```python
from build123d import *

# Parameters (mm, degrees)
CUT_EXTRUDE1_DEPTH = 101.6
SKETCH3_R          = 3.175
CUT_EXTRUDE2_DEPTH = 12.7


with BuildPart() as part:
    # Sketch1 → Revolve1 (revolve)
    with BuildSketch(Plane.XY):
        Polygon((0, 0), (27.94, 0), (27.94, 7.9375), (19.05, 7.9375), (19.05, 19.84375), (31.75, 19.84375), (31.75, 22.621875), (22.225, 22.621875), (22.225, 51.196875), (17.2640625, 51.196875), (17.2640625, 54.371875), (0, 54.371875), align=None)
    revolve(axis=Axis((0, 0, 0), (0, 1, 0)))

    # Sketch2 → Cut-Extrude1 (cut)
    with BuildSketch(Plane.XZ):
        Polygon((12.7, 7.332348419), (0, 14.664696837), (-12.7, 7.332348419), (-12.7, -7.332348419), (0, -14.664696837), (12.7, -7.332348419), align=None)
    extrude(amount=-CUT_EXTRUDE1_DEPTH, mode=Mode.SUBTRACT)

    # Sketch3 → Cut-Extrude2 (cut)
    with BuildSketch(Plane.XZ):
        with Locations((0, 22.225)):
            Circle(SKETCH3_R)
        with Locations((19.247414599, -11.1125)):
            Circle(SKETCH3_R)
        with Locations((-19.247414599, -11.1125)):
            Circle(SKETCH3_R)
    extrude(amount=-CUT_EXTRUDE2_DEPTH, mode=Mode.SUBTRACT)


solid = part.part
```
Geometry: final body of the model. Coordinates: model frame, mm. A direction names the side the tool comes from. Coordinates: 2 decimals unless noted, no trailing zeros. Order: outer loops, then holes, each group sorted by start corner. A loop starts at its lowest first (then second) coordinate and runs counter-clockwise, first axis right, second up.
Item 1: Section query D-D (z = 21). Output: boundary loops of the cut face in (x, y).
Answer:
outline: (-23.81, 19.84) - (23.81, 19.84) - (23.81, 22.62) - (7.28, 22.62) - (7.28, 51.2) - (-7.28, 51.2) - (-7.28, 22.62) - (-23.81, 22.62) - close; (-18.43, 0) - (-2.93, 0) - (-2.93, 7.94) - (-18.43, 7.94) - close; (2.93, 0) - (18.43, 0) - (18.43, 7.94) - (2.93, 7.94) - close
Item 2: Access query for faces 1 (the face through (21.199, 37.109, -6.676)), 2 (the face through (-15.12, 13.97, 11.59)), 3 (the face through (-3.64, 4.02, -27.7)), 4 (the face through (6.26, 26.81, -11.05)). Directions: +Z, -Z, +X, -X, +Y, -Y. A direction counts if a zero-diameter tool reaches every point of the face in a straight line with its end or side. Return the directions, or none.
Answer:
face 1: +Y
face 2: none
face 3: -Y
face 4: +Y, -Y
Item 3: Material intervals for line 1 along Y through (x, z) = (-24.5, -1); line 2 along Y through (x, z) = (-20, -7.5); line 3 along Z through (x, y) = (0, 35) (3 decimals), sorted ascending.
Answer:
line 1: y = 0 to 7.94, 19.84 to 22.62
line 2: y = 0 to 7.94, 19.84 to 51.2
line 3: z = -22.225 to -14.665, 14.665 to 22.225
Item 4: Contact query for flat-ended pins moving along their axis: P1, Ø6, axis at y = 15.5, z = 22.5, coming from the +X side; P2, Ø12, axis at x = 1.5, y = 23, coming from the -Z side; P3, Ø10, axis at y = 15, z = 1.5, coming from the +X side; P4, Ø1.5, axis at x = -12.5, z = 22.5, coming from the -Y side. Output: stop coordinate, or through.
Answer:
P1: passes through
P2: stops at z = -31.75
P3: stops at x = 31.75
P4: stops at y = 0
Item 5: Section query A-A (y = 15). Output: boundary loops of the cut face in (x, z).
Answer:
outline: circle Ø38.1 at (0, 0); hole (-12.7, -7.33) - (0, -14.66) - (12.7, -7.33) - (12.7, 7.33) - (0, 14.66) - (-12.7, 7.33) - close
Item 6: Section query C-C (x = 24.5). Output: boundary loops of the cut face in (y, z), then the cut area to 3 significant figures.
Answer:
outline: (0, -13.43) - (7.94, -13.43) - (7.94, 13.43) - (0, 13.43) - close; (19.84, -20.19) - (22.62, -20.19) - (22.62, 20.19) - (19.84, 20.19) - close
area: 325 mm2
Item 7: Draft query along Y for faces 5 (the face through (-6.439, 26.805, -10.947)), 6 (the face through (13, 54.372, 0)), 7 (the face through (-7, 7.938, 18)), 8 (the face through (13, 0, 0)). Return one class per face: released by +Y, released by -Y, zero draft, split by the parting line, or undercut.
Answer:
face 5: zero draft
face 6: released by +Y
face 7: undercut
face 8: released by -Y
